```python
from build123d import *

# Parameters (mm, degrees)
SKETCH3_R = 0.15


with BuildPart() as part:
    # Sweep1: sweep along a path in Sketch4
    with BuildLine(Plane(origin=(0, 0, 0), x_dir=(0, 0, -1), z_dir=(1, 0, 0))) as sweep1_path:
        Line((0, -6.5), (-5, -6.5))
        ThreePointArc((-5, -6.5), (-5.848528137, -6.148528137), (-6.2, -5.3))
        Line((-6.2, -5.3), (-6.2, -2.3))
    # Sketch3 → Sweep1 (sweep)
    with BuildSketch(Plane.XY):
        with Locations((0, -6.5)):
            Circle(SKETCH3_R)
    sweep(path=sweep1_path.line)

    # Sketch6 → Revolve1 (revolve)
    with BuildSketch(Plane(origin=(0, 0, 0), x_dir=(0, 0, -1), z_dir=(1, 0, 0)), mode=Mode.PRIVATE) as revolve1_sk:
        with BuildLine():
            Line((-6.2, -4.5), (-6.2, -2.7))
            ThreePointArc((-6.2, -2.7), (-6.193121719, -2.663553527), (-6.173433093, -2.632120836))
            Line((-6.173433093, -2.632120836), (-4.404673955, -0.718640373))
            ThreePointArc((-4.404673955, -0.718640373), (-4.371316313, -0.69490099), (-4.331240862, -0.686519537))
            Line((-4.331240862, -0.686519537), (-4.031240862, -0.686519537))
            ThreePointArc((-4.031240862, -0.686519537), (-3.960530184, -0.657230215), (-3.931240862, -0.586519537))
            Line((-3.931240862, -0.586519537), (-3.931240862, 0))
            Line((-3.931240862, 0), (-3.831240862, 0))
            Line((-3.831240862, 0), (-3.831240862, -0.586519537))
            ThreePointArc((-3.831240862, -0.586519537), (-3.889819506, -0.727940893), (-4.031240862, -0.786519537))
            Line((-4.031240862, -0.786519537), (-4.331240862, -0.786519537))
            Line((-4.331240862, -0.786519537), (-6.1, -2.7))
            Line((-6.1, -2.7), (-6.1, -4.5))
            Line((-6.1, -4.5), (-6.2, -4.5))
        make_face()
    revolve(revolve1_sk.sketch.rotate(Axis((0, 0, 6.2), (0, 0, -1)), 270), axis=Axis((0, 0, 6.2), (0, 0, -1)))


solid = part.part
```
CAD build for the part. Positions are in the model's coordinates, mm. Give positions to 0.01 mm unless a question says otherwise; leave off trailing zeros. Order: outer loops, then holes, each group sorted by start corner. A loop starts at its lowest first (then second) coordinate and runs counter-clockwise, first axis right, second up. Notation, with made-up numbers: M 62,-2.5 L 90,-2.5 A13 ccw 90,20.5 Z; hole C -11.5,-38 d8. An arc over 180 degrees is marked long. Put each result on its own line as item: value. Start each with the question number.
(1) Saw through at B-B, the plane z = 0.5. Write the cut outline in (x, y).
(2) Saw through at A-A, the plane y = 0. Write the cut outline in (x, z).
(3) Saw through at D-D, the plane z = 5.75. Give the number of separate pieces and of enclosed holes in the cut face, then the cut area to 3 significant figures.
(4) Saw through at C-C, the plane x = 4.25. Write the cut outline in (y, z), then the cut area to 3 significant figures.
(5) Flat gauge pins, fed straight in: pin 1 Ø1.5 at (y, z) = (1.5, 5) entering from +X; pin 2 Ø3 at (x, y) = (1, 1.5) entering from +Z; pin 3 Ø0.6 at (x, y) = (0, 0) entering from +Z. Where does each tip first touch, or does it go through?
(6) Drill centre lines: line 1 along X through (y, z) = (-1, 5.75); line 2 along Y through (x, z) = (-1.5, 6). Where is each one in solid material? Low to high.
Check result:
1. outline: C 0,-6.5 d0.3
2. outline: M -4.5,6.1 L -2.7,6.1 L -0.79,4.33 L -0.79,4.03 A0.2 ccw -0.59,3.83 L 0.59,3.83 A0.2 ccw 0.79,4.03 L 0.79,4.33 L 2.7,6.1 L 4.5,6.1 L 4.5,6.2 L 2.7,6.2 A0.1 ccw 2.63,6.17 L 0.72,4.4 A0.1 ccw 0.69,4.33 L 0.69,4.03 A0.1 cw 0.59,3.93 L -0.59,3.93 A0.1 cw -0.69,4.03 L -0.69,4.33 A0.1 ccw -0.72,4.4 L -2.63,6.17 A0.1 ccw -2.7,6.2 L -4.5,6.2 Z
3. separate pieces: 2
3. enclosed holes: 1
3. area: 2.17 mm2
4. outline: M -1.48,6.1 L 1.48,6.1 L 1.48,6.2 L -1.48,6.2 Z
4. area: 0.296 mm2
5. pin 1: stops at x = 1.91
5. pin 2: stops at z = 6.2
5. pin 3: stops at z = 3.93
6. line 1: x = -2.09 to -1.93, 1.93 to 2.09
6. line 2: y = -2.11 to -1.93, 1.93 to 2.11
